from build123d import *

# Parameters (mm, degrees)
SALIENTE_EXTRUIR2_DEPTH          = 50
TALADRO_DE_MARGEN_PARA_M82_D     = 9
TALADRO_DE_MARGEN_PARA_M82_DEPTH = 10
TALADRO_DE_MARGEN_PARA_M82_TIP   = 2.703872786


with BuildPart() as part:
    # Croquis3 → Saliente-Extruir2 (new, symmetric)
    with BuildSketch(Plane.XY):
        Polygon((0, 0), (0, 20), (-1, 20.577350269), (-1, 0.577350269), align=None)
    extrude(amount=SALIENTE_EXTRUIR2_DEPTH, both=True)

    # Taladro de margen para M82
    with Locations(Plane(origin=(-1, 10.577350269, -22), x_dir=(0, -1, 0), z_dir=(-1, 0, 0))):
        with Locations((0, 0), (0, 44)):
            Hole(TALADRO_DE_MARGEN_PARA_M82_D / 2, depth=TALADRO_DE_MARGEN_PARA_M82_DEPTH)
            with Locations((0, 0, -(TALADRO_DE_MARGEN_PARA_M82_DEPTH + TALADRO_DE_MARGEN_PARA_M82_TIP / 2))):  # 118° drill point
                Cone(0, TALADRO_DE_MARGEN_PARA_M82_D / 2, TALADRO_DE_MARGEN_PARA_M82_TIP, mode=Mode.SUBTRACT)


solid = part.part
Here's how the part is built. I have some questions about the finished solid (model axes, mm). Coordinates: 2 decimals unless noted, no trailing zeros. Order: outer loops, then holes, each group sorted by start corner. A loop starts at its lowest first (then second) coordinate and runs counter-clockwise, first axis right, second up.
Item 1: If we mould it in two halves opening along Y, with no side actions, what happens to faces 1 (the face through (-1, 11, 1)), 2 (the face through (-0.49, 7.26, 25.04))? For each: +Y half, -Y half, draft (parallel to the pull), parting line (faces both ways), or undercut.
Result sheet:
face 1: draft
face 2: undercut
Item 2: If we section it at A-A on z = -22: List the corners of the cut face in (x, y) for me, plus the area to 3 significant figures.
Result sheet:
outline: (-1, 0.58) - (0, 0) - (0, 6.08) - (-1, 6.08) - close; (-1, 15.08) - (0, 15.08) - (0, 20) - (-1, 20.58) - close
area: 11.0 mm2
Item 3: If we section it at C-C on x = -0.15: List the corners of the cut face in (y, z) for me.
Result sheet:
outline: (0.09, -50) - (20.09, -50) - (20.09, 50) - (0.09, 50) - close; hole circle Ø9 at (10.58, -22); hole circle Ø9 at (10.58, 22)
Item 4: If we section it at D-D on z = 3: List the corners of the cut face in (x, y) for me.
Result sheet:
outline: (-1, 0.58) - (0, 0) - (0, 20) - (-1, 20.58) - close
Item 5: If we section it at B-B on y = 14: List the corners of the cut face in (x, z) for me, plus the area to 3 significant figures.
Result sheet:
outline: (-1, -50) - (0, -50) - (0, -24.92) - (-1, -24.92) - close; (-1, -19.08) - (0, -19.08) - (0, 19.08) - (-1, 19.08) - close; (-1, 24.92) - (0, 24.92) - (0, 50) - (-1, 50) - close
area: 88.3 mm2
Item 6: I need wall thicknesses on line 1 (Z direction, x = -0.3, y = 11); line 2 (Z direction, x = -0.2, y = 14.5); line 3 (Y direction, x = -0.45, z = 23). Which ranges of each line are inside material? Lowest first, please.
Result sheet:
line 1: z = -50 to -26.48, -17.52 to 17.52, 26.48 to 50
line 2: z = -50 to -24.21, -19.79 to 19.79, 24.21 to 50
line 3: y = 0.26 to 6.19, 14.96 to 20.26
